Verification items for the finished model (mm, model axes). Round coordinates to 2 decimals unless told otherwise and drop trailing zeros. Order: outer loops, then holes, each group sorted by start corner. A loop starts at its lowest first (then second) coordinate and runs counter-clockwise, first axis right, second up. Notation, with made-up numbers: M 29,-33 L 51,-33 A14 cw 51,-13 Z; hole C -12.75,-9.5 d5. An arc over 180 degrees is marked long. Return JSON: item names as keys, results as strings. Group by question number.
Autodesk Inventor part; units mm, degrees
ref_plane "YZ Plane" through (0, 0, 0) normal (1, 0, 0) x (0, 1, 0)
ref_plane "XZ Plane" through (0, 0, 0) normal (0, 1, 0) x (-1, 0, 0)
ref_plane "XY Plane" through (0, 0, 0) normal (0, 0, 1) x (1, 0, 0)
sketch "Sketch1" plane through (0, 0, 0) normal (0, 1, 0) x (-1, 0, 0)
  circle A0 centre (0, 0) radius 33.3375
  dimension "d0" = 66.675
extrude "Extrusion1" add sketch "Sketch1" along normal blind 12.7
sketch "Sketch2" plane through (0, 12.7, 0) normal (0, 1, 0) x (1, 0, 0)
  line L0 (0, 0) -> (-3.175, 0)
  line L1 (-3.175, 0) -> (-3.175, 3.175)
  line L2 (-3.175, 3.175) -> (0, 3.175)
  line L3 (0, 3.175) -> (0, 0)
  dimension "d3" = 3.175
  dimension "d4" = 3.175
extrude "Extrusion2" cut sketch "Sketch2" against normal blind 12.7
sketch "Sketch3" plane through (0, 12.7, -3.175) normal (-1, 0, 0) x (0, 0, 1)
  line L0 (36.5125, 0) -> (-30.1625, 0)
  line L1 (36.5125, -12.7) -> (-30.1625, -12.7)
  line L2 (0, 0) -> (0, -12.7)
  line L3 (3.175, 0) -> (3.175, -12.7)
  line L4 (3.175, 0) -> (-47.625, 0)
  line L5 (-30.1625, 0) -> (-47.625, 17.4625)
  line L6 (-30.1625, 0) -> (-5.4668, 0) construction
  line L7 (-47.625, 17.4625) -> (-47.625, -12.7)
  line L8 (36.5125, 0) -> (-30.1625, 0)
  line L9 (-47.625, -12.7) -> (-30.1625, -12.7)
  line L10 (-30.1625, 0) -> (-30.1625, -12.7)
  line L11 (-30.1625, -12.7) -> (-30.1625, 0)
  line L12 (0, 0) -> (0, 32.402)
  dimension "d8" = 50.8
  dimension "d9" = 135
revolve "Revolution1" add sketch "Sketch3" angle 360 about axis through (0, 12.7, -3.175) along (0, 1, 0) contours L10 L9 L7 L4 | L4 L7 L5
fillet "Fillet1" radius 3.175 1 edges at (0, 30.1625, 44.45)
sketch "Sketch4" plane through (0, 12.7, -3.175) normal (0, 1, 0) x (1, 0, 0)
  line L0 (0, 0) -> (-3.175, 0)
  circle A0 centre (0, 0) radius 4.4901
  point P0 (0, -3.175)
extrude "Extrusion3" cut sketch "Sketch4" against normal blind 12.7
1. Go/stop test with flat-tipped pins: pin 1 (8 mm diameter, centred on x = 17.5, y = 21.5, fed in from -Z); pin 2 (12 mm diameter, centred on x = 10, z = -25.5, fed in from +Y); pin 3 (2 mm diameter, centred on x = -9.5, y = 20.5, fed in from -Z). Record where each tip stops, or that it passes through.
2. Cross-section at A-A (y = 2.25). Enter the section's corners in (x, z) (3 decimals).
3. Draft check along X on faces 1 (the face through (-0.97, 6.44, 1.21)), 2 (the face through (-10, 0, -3)), 3 (the face through (-46.492, 11.091, 7.149)). Enter one of: +X half, -X half, draft (parallel to the pull), parting line (faces both ways), or undercut.
4. Thickness scan on line 1 along Z through (x, y) = (0, 6.5); line 2 along X through (y, z) = (16.75, -12); line 3 along X through (y, z) = (16.5, -3). Record the ranges inside material, lowest first. Write a range as from..to.
Computed:
{
 "1": {"pin 1": "stops at z = -48.85", "pin 2": "stops at y = 13", "pin 3": "stops at z = -50.04"},
 "2": {"outline": "C 0,-3.175 d95.25; hole C 0,-3.175 d8.98"},
 "3": {"face 1": "undercut", "face 2": "draft", "face 3": "parting line"},
 "4": {"line 1": "z = -50.8..-7.67, 1.32..44.45", "line 2": "x = -46.8..-33.05, 33.05..46.8", "line 3": "x = -47.62..-33.96, 33.96..47.62"}
}
